Input: dimensioned drawing with shaded views. Units: mm. Origin: part minimum x, y, z. Round coordinates to 2 decimals unless told otherwise and drop trailing zeros. Loops run counter-clockwise (first coordinate to the right, second up) from the corner with the lowest first, then second, coordinate; pieces in that order, holes last. Notation, with made-up numbers: M 48,-3.5 L 59,-3.5 A11 ccw 59,4.5 Z; hole C 54,14.5 d11. An arc over 180 degrees is marked long. One line per item, written item: value.
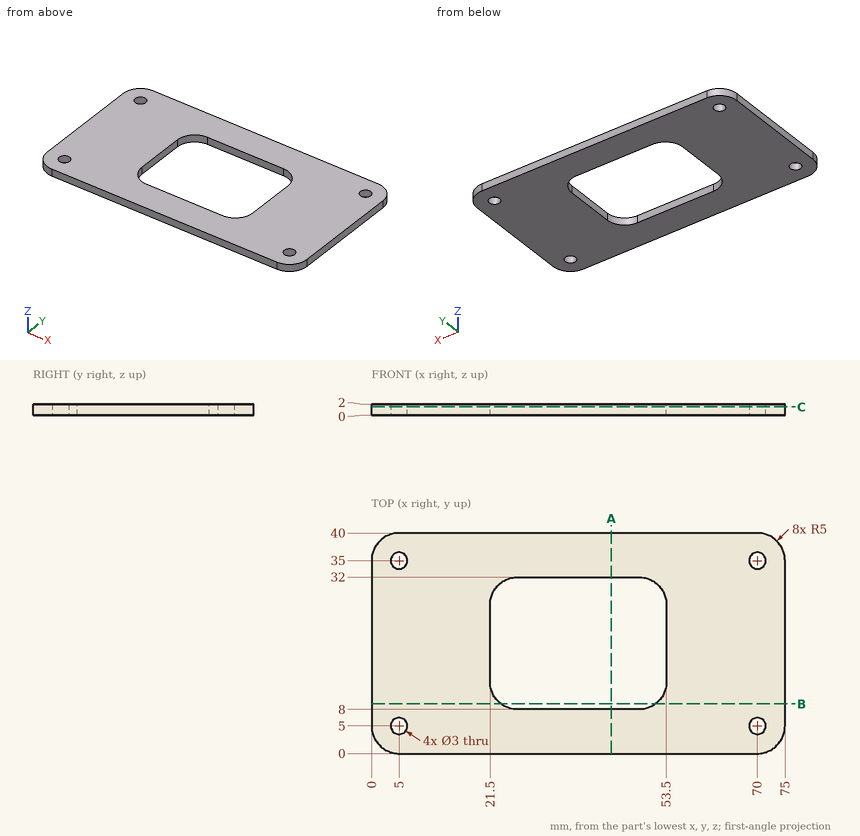
1. Section query A-A (x = 43.5). Return the cut outline in (y, z).
Report:
outline: M 0,0 L 8,0 L 8,2 L 0,2 Z; M 32,0 L 40,0 L 40,2 L 32,2 Z
2. Ray query, line 1 (Y direction, x = 5, z = 0.95); line 2 (X direction, y = 20, z = 1.95); line 3 (Y direction, x = 70.5, z = 1.85). Return the intervals inside material, ascending. Write a range as [from, to].
Report:
line 1: y = [0, 3.5], [6.5, 33.5], [36.5, 40]
line 2: x = [0, 21.5], [53.5, 75]
line 3: y = [0.03, 3.59], [6.41, 33.59], [36.41, 39.97]
3. Section query C-C (z = 1.5). Return the cut outline in (x, y).
Report:
outline: M 0,5 A5 ccw 5,0 L 70,0 A5 ccw 75,5 L 75,35 A5 ccw 70,40 L 5,40 A5 ccw 0,35 Z; hole C 5,5 d3; hole C 5,35 d3; hole M 21.5,13 A5 ccw 26.5,8 L 48.5,8 A5 ccw 53.5,13 L 53.5,27 A5 ccw 48.5,32 L 26.5,32 A5 ccw 21.5,27 Z; hole C 70,5 d3; hole C 70,35 d3
4. Section query B-B (y = 9). Return the cut outline in (x, z).
Report:
outline: M 0,0 L 23.5,0 L 23.5,2 L 0,2 Z; M 51.5,0 L 75,0 L 75,2 L 51.5,2 Z
5. Pin query (flat end, axial travel): pin 1 (1 mm diameter, centred on x = 39.5, z = 1, fed in from -Y). Return the tip coordinate at first contact, or that it passes through.
Report:
pin 1: stops at y = 0
